from build123d import *

# Parameters (mm, degrees)
SKETCH1_R           = 2.2479
SKETCH1_R_2         = 1.1
BOSS_EXTRUDE1_DEPTH = 3.175
BOSS_EXTRUDE2_START = -5.08
SKETCH1_4_R         = 2.2
SKETCH1_4_R_2       = 1.1
BOSS_EXTRUDE2_DEPTH = 5.08
SKETCH1_5_R         = 4.7879
SKETCH1_5_R_2       = 2.2479
BOSS_EXTRUDE3_DEPTH = 20.0025


with BuildPart() as part:
    # Sketch1 → Boss-Extrude1 (new body)
    with BuildSketch(Plane.XY):
        with BuildLine():
            Line((-16.612553398, 47.733487864), (-16.612553398, 6.509287864))
            ThreePointArc((-16.612553398, 6.509287864), (-15.210209956, 3.123731306), (-11.824653398, 1.721387864))
            Line((-11.824653398, 1.721387864), (37.654546627, 1.721387864))
            ThreePointArc((37.654546627, 1.721387864), (41.040103169, 3.123731315), (42.442446602, 6.509287864))
            Line((42.442446602, 6.509287864), (42.442446602, 47.733487864))
            ThreePointArc((42.442446602, 47.733487864), (41.04010316, 51.119044422), (37.654546602, 52.521387864))
            Line((37.654546602, 52.521387864), (-11.824653398, 52.521387864))
            ThreePointArc((-11.824653398, 52.521387864), (-15.210209956, 51.119044422), (-16.612553398, 47.733487864))
        make_face()
        with Locations((12.914946602, 14.421387864)):
            Circle(SKETCH1_R, mode=Mode.SUBTRACT)
        with Locations((12.914946602, 39.821387864)):
            Circle(SKETCH1_R, mode=Mode.SUBTRACT)
        with Locations((-11.824653398, 6.509287864)):
            Circle(SKETCH1_R, mode=Mode.SUBTRACT)
        with Locations((37.654546602, 6.509287864)):
            Circle(SKETCH1_R, mode=Mode.SUBTRACT)
        with Locations((-11.824653398, 47.733487864)):
            Circle(SKETCH1_R, mode=Mode.SUBTRACT)
        with Locations((37.654546602, 47.733487864)):
            Circle(SKETCH1_R, mode=Mode.SUBTRACT)
        with Locations((19.164946602, 16.621387864)):
            Circle(SKETCH1_R_2, mode=Mode.SUBTRACT)
        with Locations((6.664946602, 16.621387864)):
            Circle(SKETCH1_R_2, mode=Mode.SUBTRACT)
        with Locations((6.664946602, 37.621387864)):
            Circle(SKETCH1_R_2, mode=Mode.SUBTRACT)
        with Locations((19.164946602, 37.621387864)):
            Circle(SKETCH1_R_2, mode=Mode.SUBTRACT)
    extrude(amount=BOSS_EXTRUDE1_DEPTH)

    # Sketch1_4 → Boss-Extrude2 (add)
    # profile 1 of 4: a face of its own
    with BuildSketch(Plane.XY.offset(BOSS_EXTRUDE2_START)):
        with Locations((19.164946602, 37.621387864)):
            Circle(SKETCH1_4_R)
        with Locations((19.164946602, 37.621387864)):
            Circle(SKETCH1_4_R_2, mode=Mode.SUBTRACT)
    # profile 2 of 4: a face of its own
    with BuildSketch(Plane.XY.offset(BOSS_EXTRUDE2_START)):
        with Locations((6.664946602, 37.621387864)):
            Circle(SKETCH1_4_R)
        with Locations((6.664946602, 37.621387864)):
            Circle(SKETCH1_4_R_2, mode=Mode.SUBTRACT)
    # profile 3 of 4: a face of its own
    with BuildSketch(Plane.XY.offset(BOSS_EXTRUDE2_START)):
        with Locations((6.664946602, 16.621387864)):
            Circle(SKETCH1_4_R)
        with Locations((6.664946602, 16.621387864)):
            Circle(SKETCH1_4_R_2, mode=Mode.SUBTRACT)
    # profile 4 of 4: a face of its own
    with BuildSketch(Plane.XY.offset(BOSS_EXTRUDE2_START)):
        with Locations((19.164946602, 16.621387864)):
            Circle(SKETCH1_4_R)
        with Locations((19.164946602, 16.621387864)):
            Circle(SKETCH1_4_R_2, mode=Mode.SUBTRACT)
    extrude(amount=BOSS_EXTRUDE2_DEPTH)

    # Sketch1_5 → Boss-Extrude3 (add)
    # profile 1 of 4: a face of its own
    with BuildSketch(Plane.XY):
        with Locations((37.654546602, 47.733487864)):
            Circle(SKETCH1_5_R)
        with Locations((37.654546602, 47.733487864)):
            Circle(SKETCH1_5_R_2, mode=Mode.SUBTRACT)
    # profile 2 of 4: a face of its own
    with BuildSketch(Plane.XY):
        with Locations(Location((-11.824653398, 47.733487864, 0), (0, 0, 180))):
            Circle(SKETCH1_5_R)
        with Locations((-11.824653398, 47.733487864)):
            Circle(SKETCH1_5_R_2, mode=Mode.SUBTRACT)
    # profile 3 of 4: a face of its own
    with BuildSketch(Plane.XY):
        with Locations(Location((-11.824653398, 6.509287864, 0), (0, 0, 180))):
            Circle(SKETCH1_5_R)
        with Locations((-11.824653398, 6.509287864)):
            Circle(SKETCH1_5_R_2, mode=Mode.SUBTRACT)
    # profile 4 of 4: a face of its own
    with BuildSketch(Plane.XY):
        with Locations((37.654546602, 6.509287864)):
            Circle(SKETCH1_5_R)
        with Locations((37.654546602, 6.509287864)):
            Circle(SKETCH1_5_R_2, mode=Mode.SUBTRACT)
    extrude(amount=BOSS_EXTRUDE3_DEPTH)


solid = part.part
Geometry: final body of the model. Coordinates: model frame, mm. A direction names the side the tool comes from. Coordinates: 2 decimals unless noted, no trailing zeros. Order: outer loops, then holes, each group sorted by start corner. A loop starts at its lowest first (then second) coordinate and runs counter-clockwise, first axis right, second up.
(1) Section query B-B (y = 7.5). State how many separate pieces and enclosed holes the cut face has, plus the area to 3 significant figures.
(2) Material intervals for probe 1 along X at (y, z) = (43.5, 14.25); probe 2 along Y at (x, z) = (39.5, 18.75); probe 3 along X at (y, z) = (5.5, 8.75), sorted ascending.
(3) Draft query along X for faces 1 (the face through (42.442, 27, 2)), 2 (the face through (6.52, 17.71, -1.01)), 3 (the face through (40, 47, 20.002)), 4 (the face through (6.188, 35.474, -2.576)). Return one class per face: pulls with the +X half, pulls with the -X half, needs draft (parallel to the pull), parting line crosses it, or undercut.
(4) Section query A-A (z = 15). Return the cut outline in (x, y), plus the area to 3 significant figures.
(5) Access query for faces 5 (the face through (-14.399, 2.472, 9.861)), 6 (the face through (21.197, 15.779, -2.576)), 7 (the face through (18, 16, -5.08)). Directions: +Z, -Z, +X, -X, +Y, -Y. A direction counts if a zero-diameter tool reaches every point of the face in a straight line with its end or side. Return the directions, or none.
(6) First-contact query: pin 1 (2.5 mm diameter, centred on x = 19.16, y = 37.62, fed in from +Z) (3 decimals); pin 2 (7 mm diameter, centred on x = -11.82, y = 6.51, fed in from -Z); pin 3 (1.5 mm diameter, centred on y = 46, z = 12, fed in from +X). Flat tips, straight axial feed; report the tip coordinate or a pass-through.
(7) Section query D-D (y = 48.5). Return the cut outline in (x, z) (1 decimal), plus the area to 3 significant figures.
Solution:
1. separate pieces: 3
1. enclosed holes: 0
1. area: 341 mm2
2. probe 1: x = -14.06 to -9.59, 35.42 to 39.89
2. probe 2: y = 2.09 to 5.23, 7.79 to 10.93, 43.32 to 46.45, 49.02 to 52.15
2. probe 3: x = -16.5 to -13.83, -9.82 to -7.14, 32.97 to 35.65, 39.66 to 42.33
3. face 1: pulls with the +X half
3. face 2: undercut
3. face 3: needs draft
3. face 4: undercut
4. outline: circle Ø9.58 at (-11.82, 6.51); circle Ø9.58 at (-11.82, 47.73); circle Ø9.58 at (37.65, 6.51); circle Ø9.58 at (37.65, 47.73); hole circle Ø4.5 at (-11.82, 6.51); hole circle Ø4.5 at (-11.82, 47.73); hole circle Ø4.5 at (37.65, 6.51); hole circle Ø4.5 at (37.65, 47.73)
4. area: 225 mm2
5. face 5: +Z
5. face 6: -Z
5. face 7: -Z, +X, -X, +Y, -Y
6. pin 1: stops at z = 3.175
6. pin 2: stops at z = 0
6. pin 3: stops at x = 42.34
7. outline: (-16.6, 0) - (-13.9, 0) - (-13.9, 20) - (-16.6, 20) - close; (-9.7, 0) - (35.5, 0) - (35.5, 20) - (32.9, 20) - (32.9, 3.2) - (-7.1, 3.2) - (-7.1, 20) - (-9.7, 20) - close; (39.8, 0) - (42.4, 0) - (42.4, 20) - (39.8, 20) - close
7. area: 336 mm2
